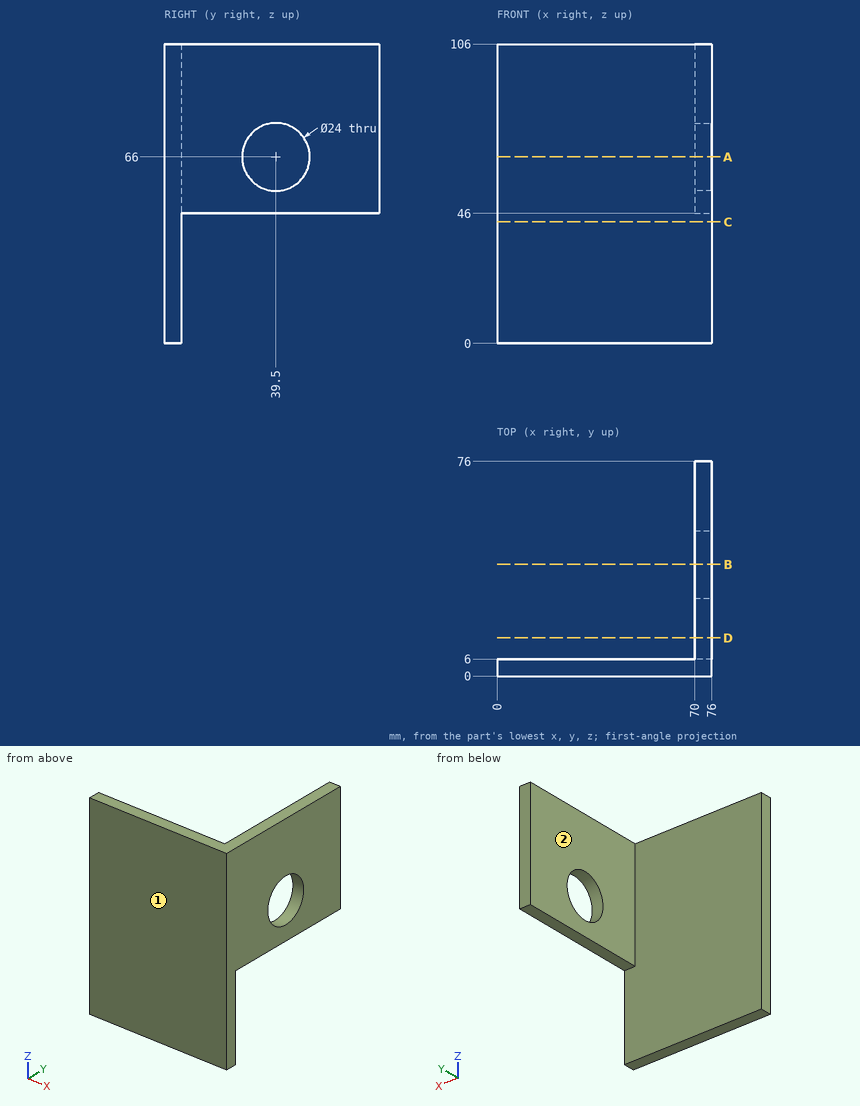
Check sheet for the drawn part. Datum: minimum x, y, z corner. Units: mm. A direction names the side the tool comes from. Round coordinates to 2 decimals unless told otherwise and drop trailing zeros. Order: outer loops, then holes, each group sorted by start corner. A loop starts at its lowest first (then second) coordinate and runs counter-clockwise, first axis right, second up. Notation, with made-up numbers: (36.25, 9) - (94.25, 9) arc R19 ccw to (94.25, 25) - close; hole circle Ø7 at (85, -9.75). An arc over 180 degrees is marked (long way). Use a Markdown table: item, result. Add a question column.
(1) Tool access check on the marked faces 1 and 2. Record the directions out of +Z, -Z, +X, -X, +Y, -Y that give a thin tool (end or side, any length) a straight path to the whole face; none if there is none.
(2) Depth check by flat-ended pin: pin 1 (1 mm diameter, centred on x = 36, z = 52.5, fed in from -Y); pin 2 (5 mm diameter, centred on x = 49.5, z = 34, fed in from +Y); pin 3 (5 mm diameter, centred on x = 71.5, y = 48, fed in from -Z); pin 4 (8 mm diameter, centred on y = 30.5, z = 60, fed in from -X). Enter the tip coordinate at first touch or a pass-through.
(3) Sectioned sample at D-D, the plane y = 13.5. Enter the section's corners in (x, z), and give its area (3 significant figures).
(4) Sectioned sample at A-A, the plane z = 66. Enter the section's corners in (x, y).
(5) Material ranges on line 1 along Y through (x, z) = (73.45, 66); line 2 along X through (y, z) = (7, 51.5); line 3 along Y through (x, z) = (68, 23.5), recorded low to high. Write a range as [from, to].
(6) Sectioned sample at C-C, the plane z = 43. Enter the section's corners in (x, y), and give its area (3 significant figures).
(7) Sectioned sample at B-B, the plane y = 39.5. Enter the section's corners in (x, z), and give its area (3 significant figures).
Answers below:
| question | item | result |
|---|---|---|
| 1 | face 1 | +Z, -Z, +X, -X, -Y |
| 1 | face 2 | +Z, -Z, -X, +Y |
| 2 | pin 1 | y = 0 |
| 2 | pin 2 | y = 6 |
| 2 | pin 3 | z = 46 |
| 2 | pin 4 | x = 70 |
| 3 | outline | (70, 46) - (76, 46) - (76, 106) - (70, 106) - close |
| 3 | area | 360 mm² |
| 4 | outline | (0, 0) - (76, 0) - (76, 27.5) - (70, 27.5) - (70, 6) - (0, 6) - close; (70, 51.5) - (76, 51.5) - (76, 76) - (70, 76) - close |
| 5 | line 1 | [0, 27.5], [51.5, 76] |
| 5 | line 2 | [70, 76] |
| 5 | line 3 | [0, 6] |
| 6 | outline | (0, 0) - (76, 0) - (76, 6) - (0, 6) - close |
| 6 | area | 456 mm² |
| 7 | outline | (70, 46) - (76, 46) - (76, 54) - (70, 54) - close; (70, 78) - (76, 78) - (76, 106) - (70, 106) - close |
| 7 | area | 216 mm² |
